Design review of the part built by this model. Coordinates are the model's own, in mm. A direction names the side the tool comes from. Coordinates: 2 decimals unless noted, no trailing zeros. Order: outer loops, then holes, each group sorted by start corner. A loop starts at its lowest first (then second) coordinate and runs counter-clockwise, first axis right, second up. Notation, with made-up numbers: M 43.25,-9 L 87.25,-9 A28 ccw 87.25,12 Z; hole C -27.5,-8 d11. An arc over 180 degrees is marked long. Answer in a Markdown table with one row per item.
from build123d import *

# Parameters (mm, degrees)
SKETCH_1_W          = 31
SKETCH_1_H          = 48
EXTRUDE_1_DEPTH     = 1.2
CUT_EXTRUDE_1_REACH = 59.153
SKETCH_2_R          = 1.05
CUT_EXTRUDE_2_REACH = 59.153
SKETCH_3_R          = 0.5
SKETCH_4_W          = 30.07
SKETCH_4_H          = 37.43
EXTRUDE_2_DEPTH     = 1.56
FILLET_1_R          = 5


with BuildPart() as part:
    # 草图1 → 凸台-拉伸1 (new body)
    with BuildSketch(Plane(origin=(0, 0, 0), x_dir=(1, 0, 0), z_dir=(0, 1, 0))):
        with Locations((15.5, -24)):
            Rectangle(SKETCH_1_W, SKETCH_1_H)
    extrude(amount=EXTRUDE_1_DEPTH)

    # 草图2 → 切除-拉伸1 (cut, up to next)
    with BuildSketch(Plane(origin=(0, 1.2, 0), x_dir=(1, 0, 0), z_dir=(0, 1, 0)), mode=Mode.PRIVATE) as cut_extrude_1_sk1:
        with Locations(Location((2.5, -2.5, 0), (0, 0, 270))):
            Circle(SKETCH_2_R)
    cut_extrude_1_tool1 = extrude(cut_extrude_1_sk1.sketch, amount=-CUT_EXTRUDE_1_REACH, mode=Mode.PRIVATE) & part.part
    # 草图2 → 切除-拉伸1 (cut, up to next)
    with BuildSketch(Plane(origin=(0, 1.2, 0), x_dir=(1, 0, 0), z_dir=(0, 1, 0)), mode=Mode.PRIVATE) as cut_extrude_1_sk2:
        with Locations(Location((28.5, -2.5, 0), (0, 0, 270))):
            Circle(SKETCH_2_R)
    cut_extrude_1_tool2 = extrude(cut_extrude_1_sk2.sketch, amount=-CUT_EXTRUDE_1_REACH, mode=Mode.PRIVATE) & part.part
    # 草图2 → 切除-拉伸1 (cut, up to next)
    with BuildSketch(Plane(origin=(0, 1.2, 0), x_dir=(1, 0, 0), z_dir=(0, 1, 0)), mode=Mode.PRIVATE) as cut_extrude_1_sk3:
        with Locations(Location((2.5, -45.5, 0), (0, 0, 270))):
            Circle(SKETCH_2_R)
    cut_extrude_1_tool3 = extrude(cut_extrude_1_sk3.sketch, amount=-CUT_EXTRUDE_1_REACH, mode=Mode.PRIVATE) & part.part
    # 草图2 → 切除-拉伸1 (cut, up to next)
    with BuildSketch(Plane(origin=(0, 1.2, 0), x_dir=(1, 0, 0), z_dir=(0, 1, 0)), mode=Mode.PRIVATE) as cut_extrude_1_sk4:
        with Locations(Location((28.5, -45.5, 0), (0, 0, 270))):
            Circle(SKETCH_2_R)
    cut_extrude_1_tool4 = extrude(cut_extrude_1_sk4.sketch, amount=-CUT_EXTRUDE_1_REACH, mode=Mode.PRIVATE) & part.part
    add(cut_extrude_1_tool1.solids().sort_by_distance((2.5, 1.2, 2.5))[0], mode=Mode.SUBTRACT)
    add(cut_extrude_1_tool2.solids().sort_by_distance((28.5, 1.2, 2.5))[0], mode=Mode.SUBTRACT)
    add(cut_extrude_1_tool3.solids().sort_by_distance((2.5, 1.2, 45.5))[0], mode=Mode.SUBTRACT)
    add(cut_extrude_1_tool4.solids().sort_by_distance((28.5, 1.2, 45.5))[0], mode=Mode.SUBTRACT)

    # 草图3 → 切除-拉伸2 (cut, up to next)
    with BuildSketch(Plane(origin=(0, 1.2, 0), x_dir=(1, 0, 0), z_dir=(0, 1, 0)), mode=Mode.PRIVATE) as cut_extrude_2_sk1:
        with Locations(Location((14.23, -1.5, 0), (0, 0, 270))):
            Circle(SKETCH_3_R)
    cut_extrude_2_tool1 = extrude(cut_extrude_2_sk1.sketch, amount=-CUT_EXTRUDE_2_REACH, mode=Mode.PRIVATE) & part.part
    # 草图3 → 切除-拉伸2 (cut, up to next)
    with BuildSketch(Plane(origin=(0, 1.2, 0), x_dir=(1, 0, 0), z_dir=(0, 1, 0)), mode=Mode.PRIVATE) as cut_extrude_2_sk2:
        with Locations(Location((11.69, -1.5, 0), (0, 0, 270))):
            Circle(SKETCH_3_R)
    cut_extrude_2_tool2 = extrude(cut_extrude_2_sk2.sketch, amount=-CUT_EXTRUDE_2_REACH, mode=Mode.PRIVATE) & part.part
    # 草图3 → 切除-拉伸2 (cut, up to next)
    with BuildSketch(Plane(origin=(0, 1.2, 0), x_dir=(1, 0, 0), z_dir=(0, 1, 0)), mode=Mode.PRIVATE) as cut_extrude_2_sk3:
        with Locations(Location((9.15, -1.5, 0), (0, 0, 270))):
            Circle(SKETCH_3_R)
    cut_extrude_2_tool3 = extrude(cut_extrude_2_sk3.sketch, amount=-CUT_EXTRUDE_2_REACH, mode=Mode.PRIVATE) & part.part
    # 草图3 → 切除-拉伸2 (cut, up to next)
    with BuildSketch(Plane(origin=(0, 1.2, 0), x_dir=(1, 0, 0), z_dir=(0, 1, 0)), mode=Mode.PRIVATE) as cut_extrude_2_sk4:
        with Locations(Location((6.61, -1.5, 0), (0, 0, 270))):
            Circle(SKETCH_3_R)
    cut_extrude_2_tool4 = extrude(cut_extrude_2_sk4.sketch, amount=-CUT_EXTRUDE_2_REACH, mode=Mode.PRIVATE) & part.part
    # 草图3 → 切除-拉伸2 (cut, up to next)
    with BuildSketch(Plane(origin=(0, 1.2, 0), x_dir=(1, 0, 0), z_dir=(0, 1, 0)), mode=Mode.PRIVATE) as cut_extrude_2_sk5:
        with Locations(Location((24.39, -1.5, 0), (0, 0, 270))):
            Circle(SKETCH_3_R)
    cut_extrude_2_tool5 = extrude(cut_extrude_2_sk5.sketch, amount=-CUT_EXTRUDE_2_REACH, mode=Mode.PRIVATE) & part.part
    # 草图3 → 切除-拉伸2 (cut, up to next)
    with BuildSketch(Plane(origin=(0, 1.2, 0), x_dir=(1, 0, 0), z_dir=(0, 1, 0)), mode=Mode.PRIVATE) as cut_extrude_2_sk6:
        with Locations(Location((21.85, -1.5, 0), (0, 0, 270))):
            Circle(SKETCH_3_R)
    cut_extrude_2_tool6 = extrude(cut_extrude_2_sk6.sketch, amount=-CUT_EXTRUDE_2_REACH, mode=Mode.PRIVATE) & part.part
    # 草图3 → 切除-拉伸2 (cut, up to next)
    with BuildSketch(Plane(origin=(0, 1.2, 0), x_dir=(1, 0, 0), z_dir=(0, 1, 0)), mode=Mode.PRIVATE) as cut_extrude_2_sk7:
        with Locations(Location((19.31, -1.5, 0), (0, 0, 270))):
            Circle(SKETCH_3_R)
    cut_extrude_2_tool7 = extrude(cut_extrude_2_sk7.sketch, amount=-CUT_EXTRUDE_2_REACH, mode=Mode.PRIVATE) & part.part
    # 草图3 → 切除-拉伸2 (cut, up to next)
    with BuildSketch(Plane(origin=(0, 1.2, 0), x_dir=(1, 0, 0), z_dir=(0, 1, 0)), mode=Mode.PRIVATE) as cut_extrude_2_sk8:
        with Locations(Location((16.77, -1.5, 0), (0, 0, 270))):
            Circle(SKETCH_3_R)
    cut_extrude_2_tool8 = extrude(cut_extrude_2_sk8.sketch, amount=-CUT_EXTRUDE_2_REACH, mode=Mode.PRIVATE) & part.part
    add(cut_extrude_2_tool1.solids().sort_by_distance((14.23, 1.2, 1.5))[0], mode=Mode.SUBTRACT)
    add(cut_extrude_2_tool2.solids().sort_by_distance((11.69, 1.2, 1.5))[0], mode=Mode.SUBTRACT)
    add(cut_extrude_2_tool3.solids().sort_by_distance((9.15, 1.2, 1.5))[0], mode=Mode.SUBTRACT)
    add(cut_extrude_2_tool4.solids().sort_by_distance((6.61, 1.2, 1.5))[0], mode=Mode.SUBTRACT)
    add(cut_extrude_2_tool5.solids().sort_by_distance((24.39, 1.2, 1.5))[0], mode=Mode.SUBTRACT)
    add(cut_extrude_2_tool6.solids().sort_by_distance((21.85, 1.2, 1.5))[0], mode=Mode.SUBTRACT)
    add(cut_extrude_2_tool7.solids().sort_by_distance((19.31, 1.2, 1.5))[0], mode=Mode.SUBTRACT)
    add(cut_extrude_2_tool8.solids().sort_by_distance((16.77, 1.2, 1.5))[0], mode=Mode.SUBTRACT)

    # 草图4 → 凸台-拉伸2 (add)
    with BuildSketch(Plane(origin=(0, 1.2, 0), x_dir=(1, 0, 0), z_dir=(0, 1, 0))):
        with Locations((15.5, -24)):
            Rectangle(SKETCH_4_W, SKETCH_4_H)
    extrude(amount=EXTRUDE_2_DEPTH)

    # 圆角1
    fillet_1_edges = [part.edges().sort_by_distance(p)[0] for p in [
        (0.465, 1.98, 5.285),
        (0.465, 1.98, 42.715),
        (30.535, 1.98, 42.715),
        (30.535, 1.98, 5.285),
    ]]
    fillet(fillet_1_edges, radius=FILLET_1_R)


solid = part.part
(1) Add section A-A, the plane x = 19.31. Give the boundary of the cut face in (y, z) (3 decimals), and give its area (3 significant figures).
Return value:
| item | result |
|---|---|
| outline | M 0,0 L 1.2,0 L 1.2,1 L 0,1 Z; M 0,2 L 1.2,2 L 1.2,5.285 L 2.76,5.285 L 2.76,42.715 L 1.2,42.715 L 1.2,48 L 0,48 Z |
| area | 115 mm2 |
(2) Draft analysis for pull direction X (two halves, no side actions). For faces 1 (the cylindrical face through (1.97, 1.99, 6.71)), 2 (the flat face through (15, 1, 48)), 3 (the cylindrical face through (23.9, 0.6, 1.4)), state which applies: pulls with the +X half, pulls with the -X half, needs draft (parallel to the pull), parting line crosses it, or undercut.
Return value:
| item | result |
|---|---|
| face 1 | pulls with the -X half |
| face 2 | needs draft |
| face 3 | undercut |
(3) For line 1 along X through (y, z) = (0.85, 2.5); line 2 along X through (y, z) = (0.5, 46); line 3 along X through (y, z) = (1.7, 12) (3 decimals), list the stretches that pass through material, from the lowest coordinate up. Write a range as from..to.
Return value:
| item | result |
|---|---|
| line 1 | x = 0..1.45, 3.55..27.45, 29.55..31 |
| line 2 | x = 0..1.58, 3.42..27.58, 29.42..31 |
| line 3 | x = 0.465..30.535 |
(4) For faces 4 (the flat face through (0.465, 2, 24)), 5 (the cylindrical face through (29.11, 1.99, 6.79)), 6 (the cylindrical face through (1.97, 1.99, 41.29)), list the 3-axis set-ups (+Z, -Z, +X, -X, +Y, -Y) from which the entire face can be reached by the end or side of a thin tool; tool diameter is ignored.
Return value:
| item | result |
|---|---|
| face 4 | +Z, -Z, -X, +Y |
| face 5 | -Z, +X, +Y |
| face 6 | +Z, -X, +Y |
(5) Insertion check: pin 1 Ø0.8 at (y, z) = (2, 20.5) entering from +X (3 decimals); pin 2 Ø0.8 at (y, z) = (2, 22.5) entering from -X (3 decimals); pin 3 Ø2.5 at (x, z) = (2.5, 2.5) entering from +Y; pin 4 Ø1.9 at (x, z) = (28.5, 45.5) entering from +Y. Each pin has a flat end and moves straight along its axis. Give the tip position at first contact, or say it passes through.
Return value:
| item | result |
|---|---|
| pin 1 | stops at x = 30.535 |
| pin 2 | stops at x = 0.465 |
| pin 3 | stops at y = 1.2 |
| pin 4 | passes through |
(6) Add section B-B, the plane z = 2.5. Give the boundary of the cut face in (x, y), and give its area (3 significant figures).
Return value:
| item | result |
|---|---|
| outline | M 0,0 L 1.45,0 L 1.45,1.2 L 0,1.2 Z; M 3.55,0 L 27.45,0 L 27.45,1.2 L 3.55,1.2 Z; M 29.55,0 L 31,0 L 31,1.2 L 29.55,1.2 Z |
| area | 32.2 mm2 |
(7) Add section D-D, the plane x = 15.5. Give the boundary of the cut face in (y, z) (3 decimals), and give its area (3 significant figures).
Return value:
| item | result |
|---|---|
| outline | M 0,0 L 1.2,0 L 1.2,5.285 L 2.76,5.285 L 2.76,42.715 L 1.2,42.715 L 1.2,48 L 0,48 Z |
| area | 116 mm2 |
(8) Add section C-C, the plane y = 1.7. Give the boundary of the cut face in (x, z) (3 decimals), and give its area (3 significant figures).
Return value:
| item | result |
|---|---|
| outline | M 0.465,10.285 A5 ccw 5.465,5.285 L 25.535,5.285 A5 ccw 30.535,10.285 L 30.535,37.715 A5 ccw 25.535,42.715 L 5.465,42.715 A5 ccw 0.465,37.715 Z |
| area | 1,100 mm2 |
